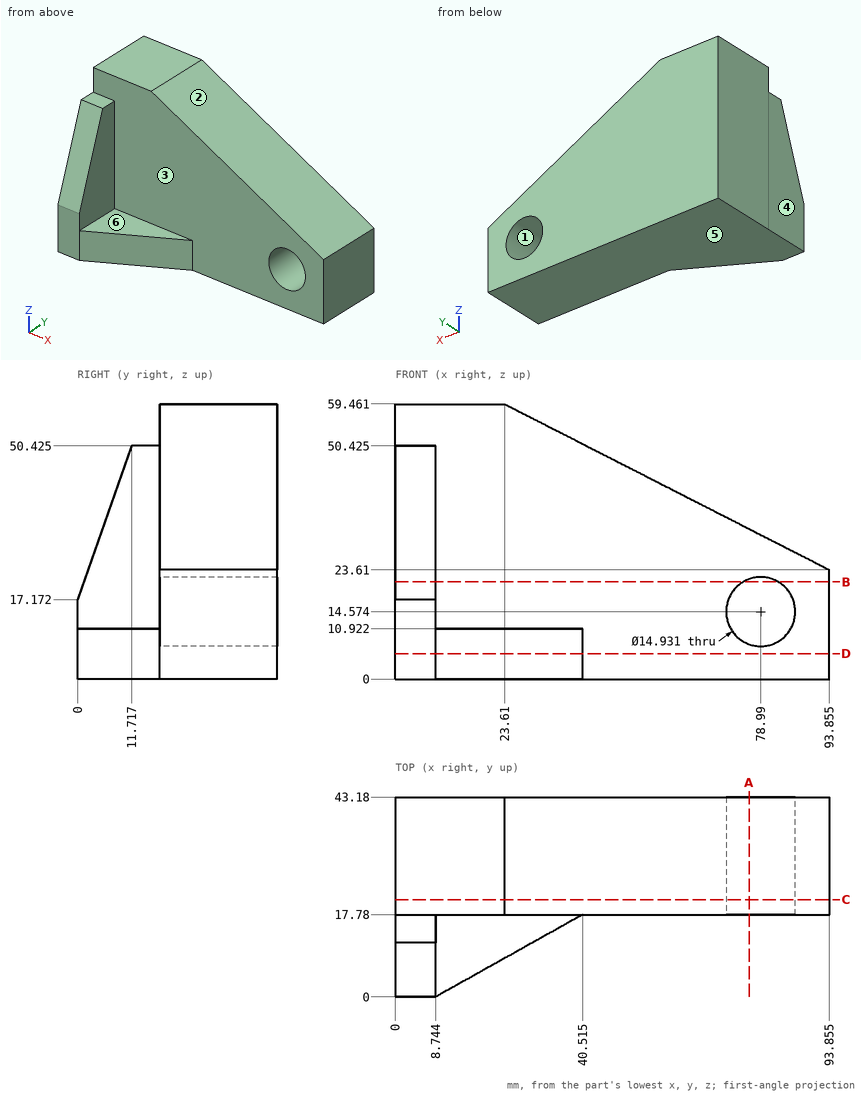
Job drawing, mm, ordinate dimensions from the low corner. One solid piece. A direction names the side the tool comes from. Round coordinates to 2 decimals unless told otherwise and drop trailing zeros. Write each loop counter-clockwise with the first axis right and the second up, starting at its lowest first coordinate (ties: lowest second). Pieces come first, ordered by that corner, then holes. Notation, with made-up numbers: M -30,51.5 L 10,51.5 A23 cw 10,70.5 Z; hole C 17,29.5 d7. An arc over 180 degrees is marked long. Return JSON: item names as keys, results as strings. Group by question number.
(1) Saw through at D-D on z = 5.5. Write the cut outline in (x, y) (1 decimal).
(2) Drill centre lines: probe 1 along Y at (x, z) = (23, 36.5); probe 2 along X at (y, z) = (25.5, 21) (1 decimal); probe 3 along X at (y, z) = (11, 12.5) (1 decimal). Where is each one in solid material? Low to high.
(3) Saw through at C-C on y = 21. Write the cut outline in (x, z) (1 decimal).
(4) Two-plate mould, pull along X, no slides. Class the marked faces 1, 2, 3 and 4: +X half, -X half, draft (parallel to the pull), parting line (faces both ways), or undercut.
(5) Saw through at A-A on x = 76.5. Write the cut outline in (y, z) (1 decimal).
(6) Saw through at B-B on z = 21. Write the cut outline in (x, y) (1 decimal).
(7) Pin check, flat tips, straight feed: pin 1 Ø1 at (x, y) = (45, 23) entering from +Z; pin 2 Ø18 at (x, z) = (30.5, 42.5) entering from -Y; pin 3 Ø1.8 at (x, y) = (6.5, 15.5) entering from +Z (1 decimal). Stop position of each tip, or through.
(8) Which spindle directions (+Z, -Z, +X, -X, +Y, -Y) get a long thin tool onto all of the face, cutting with end or side? Do the marked faces 5 and 6. Say none if no direction does.
Returned:
{
 "1": {"outline": "M 0,0 L 8.7,0 L 40.5,17.8 L 93.9,17.8 L 93.9,43.2 L 0,43.2 Z"},
 "2": {"probe 1": "17.78 to 43.18", "probe 2": "0 to 75.2, 82.8 to 93.9", "probe 3": "0 to 8.7"},
 "3": {"outline": "M 0,0 L 93.9,0 L 93.9,23.6 L 23.6,59.5 L 0,59.5 Z; hole C 79,14.6 d14.9"},
 "4": {"face 1": "undercut", "face 2": "+X half", "face 3": "draft", "face 4": "-X half"},
 "5": {"outline": "M 17.8,0 L 43.2,0 L 43.2,7.5 L 17.8,7.5 Z; M 17.8,21.6 L 43.2,21.6 L 43.2,32.5 L 17.8,32.5 Z"},
 "6": {"outline": "M 0,1.3 L 8.7,1.3 L 8.7,17.8 L 75.2,17.8 L 75.2,43.2 L 0,43.2 Z; M 82.8,17.8 L 93.9,17.8 L 93.9,43.2 L 82.8,43.2 Z"},
 "7": {"pin 1": "z = 48.8", "pin 2": "y = 17.78", "pin 3": "z = 50.4"},
 "8": {"face 5": "-Z, +X, -X, +Y, -Y", "face 6": "+Z, +X, -Y"}
}
